The model under review builds one solid part; all positions refer to its coordinate system, in mm. Face numbers are marked on the shaded views. A direction names the side the tool comes from. Give positions to 0.01 mm unless a question says otherwise; leave off trailing zeros. Loops run counter-clockwise (first coordinate to the right, second up) from the corner with the lowest first, then second, coordinate; pieces in that order, holes last. Notation, with made-up numbers: (55.5, 17) - (64.5, 17) arc R24 ccw to (64.5, 36) - close; hole circle Ø1 at (-8, 11). An arc over 180 degrees is marked (long way). Return JSON: item names as keys, results as strings. Group by question number.
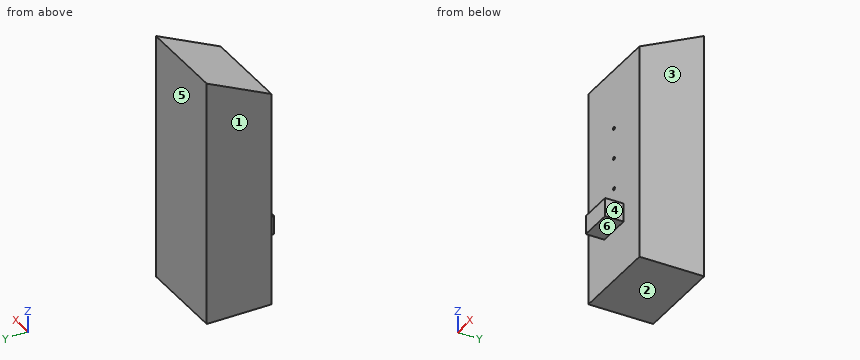
```python
from build123d import *

# Parameters (mm, degrees)
BOSS_EXTRUDE1_DEPTH             = 145
TAP_DRILL_FOR_1_4_20_TAP1_D     = 5.1054
TAP_DRILL_FOR_1_4_20_TAP1_DEPTH = 8
TAP_DRILL_FOR_1_4_20_TAP1_TIP   = 1.533816902
SKETCH4_W                       = 55
SKETCH4_H                       = 30
BOSS_EXTRUDE2_DEPTH             = 30


with BuildPart() as part:
    # Sketch1 → Boss-Extrude1 (new body)
    with BuildSketch(Plane(origin=(0, 0, 0), x_dir=(0, 0, -1), z_dir=(1, 0, 0))):
        Polygon((-350, 0), (0, 0), (0, 105), (-400, 105), align=None)
    extrude(amount=BOSS_EXTRUDE1_DEPTH)

    # Tap Drill for 1/4-20 Tap1
    with Locations(Plane(origin=(0, 0, 0), x_dir=(-1, 0, 0), z_dir=(0, -1, 0))):
        with Locations((-72.5, -253), (-72.5, -203), (-72.5, -153)):
            Hole(TAP_DRILL_FOR_1_4_20_TAP1_D / 2, depth=TAP_DRILL_FOR_1_4_20_TAP1_DEPTH)
            with Locations((0, 0, -(TAP_DRILL_FOR_1_4_20_TAP1_DEPTH + TAP_DRILL_FOR_1_4_20_TAP1_TIP / 2))):  # 118° drill point
                Cone(0, TAP_DRILL_FOR_1_4_20_TAP1_D / 2, TAP_DRILL_FOR_1_4_20_TAP1_TIP, mode=Mode.SUBTRACT)

    # Sketch4 → Boss-Extrude2 (add)
    with BuildSketch(Plane.XZ):
        with Locations((72.5, 98)):
            Rectangle(SKETCH4_W, SKETCH4_H)
    extrude(amount=BOSS_EXTRUDE2_DEPTH)


solid = part.part
```
1) We need section C-C, the plane z = 196. Write out the cut boundary in (x, y).
2) For pin 1 Ø15 at (y, z) = (-16, 98) entering from -X; pin 2 Ø9 at (y, z) = (-8, 91.5) entering from +X; pin 3 Ø1.5 at (x, y) = (98, 40) entering from +Z, all flat-tipped, find the tip position at first contact; note any pin that passes through.
3) To check wall thickness, follow line 1 (X direction, y = 3, z = 253); line 2 (Z direction, x = 72, y = 5); line 3 (Z direction, x = 72.5, y = 4.5). State the ranges of each line that lie inside material, in increasing order.
4) Tool access review of the marked faces 4, 5 and 6: name each direction out of +Z, -Z, +X, -X, +Y, -Y from which nothing blocks a thin tool from reaching the whole face with its end or side.
5) We need section B-B, the plane y = 31.5. Write out the cut boundary in (x, z), plus the area to 3 significant figures.
6) We need section A-A, the plane x = 58.5. Write out the cut boundary in (y, z), plus the area to 3 significant figures.
7) Draft analysis for pull direction X (two halves, no side actions). For the marked faces 1, 2 and 3, state which applies: +X half, -X half, draft (parallel to the pull), parting line (faces both ways), or undercut.
Findings:
{
 "1": {"outline": "(0, 0) - (145, 0) - (145, 105) - (0, 105) - close"},
 "2": {"pin 1": "stops at x = 45", "pin 2": "stops at x = 100", "pin 3": "stops at z = 369.4"},
 "3": {"line 1": "x = 0 to 69.95, 75.05 to 145", "line 2": "z = 0 to 150.5, 155.5 to 200.5, 205.5 to 250.5, 255.5 to 352.38", "line 3": "z = 0 to 150.45, 155.55 to 200.45, 205.55 to 250.45, 255.55 to 352.14"},
 "4": {"face 4": "+Z, -Z, +X, -Y", "face 5": "+Z, -Z, +X, -X, +Y", "face 6": "-Z, +X, -X, -Y"},
 "5": {"outline": "(0, 0) - (145, 0) - (145, 365) - (0, 365) - close", "area": "52,900 mm^2"},
 "6": {"outline": "(-30, 83) - (0, 83) - (0, 0) - (105, 0) - (105, 400) - (0, 350) - (0, 113) - (-30, 113) - close", "area": "40,300 mm^2"},
 "7": {"face 1": "-X half", "face 2": "draft", "face 3": "+X half"}
}
